```python
from build123d import *
from build123d.topology import SkipClean

# Parameters (mm, degrees)
BOSS_EXTRUDE1_START = 55
SKETCH2_W           = 105
SKETCH2_H           = 22
SKETCH2_R           = 1.8
BOSS_EXTRUDE1_DEPTH = 2
BOSS_EXTRUDE2_START = 2
SKETCH3_R           = 3.8
SKETCH3_R_2         = 1.8
BOSS_EXTRUDE2_DEPTH = 2
BOSS_EXTRUDE3_START = 15
SKETCH5_W           = 105
SKETCH5_H           = 22
SKETCH5_R           = 1.5
BOSS_EXTRUDE3_DEPTH = 2
SKETCH6_W           = 114
SKETCH6_H           = 2
BOSS_EXTRUDE4_DEPTH = 11


with BuildPart() as part:
    # Sketch2 → Boss-Extrude1 (new body)
    with BuildSketch(Plane(origin=(0, 0, 0), x_dir=(0, 0, -1), z_dir=(1, 0, 0)).offset(BOSS_EXTRUDE1_START)):
        Rectangle(SKETCH2_W, SKETCH2_H)
        Circle(SKETCH2_R, mode=Mode.SUBTRACT)
        with Locations((-25.5, 0)):
            Circle(SKETCH2_R, mode=Mode.SUBTRACT)
        with Locations((25.5, 0)):
            Circle(SKETCH2_R, mode=Mode.SUBTRACT)
    extrude(amount=BOSS_EXTRUDE1_DEPTH)

    # Sketch3 → Boss-Extrude2 (add)
    # profile 1 of 2: a face of its own
    with SkipClean():  # the faces are left unmerged after this step: merging them gives an invalid solid
        with BuildSketch(Plane.ZY.offset(-55).offset(BOSS_EXTRUDE2_START)):
            with Locations((-25.5, 0)):
                Circle(SKETCH3_R)
            with Locations((-25.5, 0)):
                Circle(SKETCH3_R_2, mode=Mode.SUBTRACT)
        # profile 2 of 2: a face of its own
        with BuildSketch(Plane.ZY.offset(-55).offset(BOSS_EXTRUDE2_START)):
            with Locations((25.5, 0)):
                Circle(SKETCH3_R)
            with Locations((25.5, 0)):
                Circle(SKETCH3_R_2, mode=Mode.SUBTRACT)
        extrude(amount=-BOSS_EXTRUDE2_DEPTH)


with BuildPart() as body_2:
    # Sketch5 → Boss-Extrude3 (new body)
    with BuildSketch(Plane(origin=(0, 0, 0), x_dir=(0, 0, -1), z_dir=(1, 0, 0)).offset(BOSS_EXTRUDE3_START)):
        Rectangle(SKETCH5_W, SKETCH5_H)
        with Locations((8, 0)):
            Circle(SKETCH5_R, mode=Mode.SUBTRACT)
        with Locations((-8, 0)):
            Circle(SKETCH5_R, mode=Mode.SUBTRACT)
        with Locations((0, 6)):
            Circle(SKETCH5_R, mode=Mode.SUBTRACT)
        with Locations((0, -6)):
            Circle(SKETCH5_R, mode=Mode.SUBTRACT)
    extrude(amount=BOSS_EXTRUDE3_DEPTH)


with BuildPart() as body_3:
    # Mirror2: mirrored copy
    add(part.part.mirror(Plane(origin=(0, 0, 0), x_dir=(0, 0, 1), z_dir=(1, 0, 0))))


with BuildPart() as body_4:
    # Mirror2 2: mirrored copy
    add(body_2.part.mirror(Plane(origin=(0, 0, 0), x_dir=(0, 0, 1), z_dir=(1, 0, 0))))


with BuildPart() as part_1:
    with SkipClean():  # the faces are left unmerged after this step: merging them gives an invalid solid
        add(part.part)

        add(body_2.part)  # Boss-Extrude4 merges body 2

        add(body_3.part)  # Boss-Extrude4 merges body 3

        add(body_4.part)  # Boss-Extrude4 merges body 4
        # Sketch6 → Boss-Extrude4 (add, symmetric)
        with BuildSketch(Plane(origin=(0, 0, 0), x_dir=(1, 0, 0), z_dir=(0, 1, 0))):
            with Locations((0, -51.5)):
                Rectangle(SKETCH6_W, SKETCH6_H)
            with Locations((0, 51.5)):
                Rectangle(SKETCH6_W, SKETCH6_H)
        extrude(amount=BOSS_EXTRUDE4_DEPTH, both=True)


solid = part_1.part
```
Model file for the job. Use its own axes, mm. A direction names the side the tool comes from. Coordinates: 2 decimals unless noted, no trailing zeros. Loops run counter-clockwise (first coordinate to the right, second up) from the corner with the lowest first, then second, coordinate; pieces in that order, holes last. Notation, with made-up numbers: (75.25, 11) - (120.25, 11) arc R27 ccw to (120.25, 42) - close; hole circle Ø8 at (-2.5, 8). An arc over 180 degrees is marked (long way). Answer as a JSON object with one key per item and string values. Group by question number.
(1) Cut at A-A (z = -14.5). Give the cut face in (x, y).
(2) Flat gauge pin, fed straight in: pin 1 (3 mm diameter, centred on y = 0, z = 0, fed in from -X). Where does the tip first touch, or does it go through?
(3) Cut at C-C (z = -25.5). State how many separate pieces and enclosed holes the cut face has, then the cut area to 3 significant figures.
(4) Tool access for faces 1 (the face through (15.99, 0.07, 9.5)), 2 (the face through (15, 0, 1)), 3 (the face through (-16.6, -11, 15.8)): list every direction of +Z, -Z, +X, -X, +Y, -Y with a clear straight run to the whole face (end or side of a thin tool).
(5) Probe line 1 along X through (y, z) = (-2.5, -23.5); line 2 along Y through (x, z) = (-16.25, 0); line 3 along X through (y, z) = (-6, -43). List the from-to ranges inside material, lowest first.
(6) Cut at B-B (x = 33). Give the cut face in (y, z), then the cut area to 3 significant figures.
(7) Two-plate mould, pull along X, no slides. Class faces 4 (the face through (-17, 0, 1)), 5 (the face through (-55.986, 0.541, -1.717)): released by +X, released by -X, zero draft, split by the parting line, or undercut.
(8) Cut at D-D (y = -6). Give the cut face in (x, z), then the cut area to 3 significant figures.
Geometry says:
{
 "1": {"outline": "(-57, -11) - (-55, -11) - (-55, 11) - (-57, 11) - close; (-17, -11) - (-15, -11) - (-15, 11) - (-17, 11) - close; (15, -11) - (17, -11) - (17, 11) - (15, 11) - close; (55, -11) - (57, -11) - (57, 11) - (55, 11) - close"},
 "2": {"pin 1": "stops at x = -17"},
 "3": {"separate pieces": "6", "enclosed holes": "0", "area": "178 mm^2"},
 "4": {"face 1": "none", "face 2": "+Y, -Y", "face 3": "+Z, -Z, +X, -X, -Y"},
 "5": {"line 1": "x = -57 to -53, -17 to -15, 15 to 17, 53 to 57", "line 2": "y = -11 to -7.5, -4.5 to 4.5, 7.5 to 11", "line 3": "x = -57 to -55, -17 to -15, 15 to 17, 55 to 57"},
 "6": {"outline": "(-11, -52.5) - (11, -52.5) - (11, -50.5) - (-11, -50.5) - close; (-11, 50.5) - (11, 50.5) - (11, 52.5) - (-11, 52.5) - close", "area": "88.0 mm^2"},
 "7": {"face 4": "undercut", "face 5": "zero draft"},
 "8": {"outline": "(-57, -52.5) - (57, -52.5) - (57, 52.5) - (-57, 52.5) - close; hole (-55, -50.5) - (-17, -50.5) - (-17, -1.5) - (-15, -1.5) - (-15, -50.5) - (15, -50.5) - (15, -1.5) - (17, -1.5) - (17, -50.5) - (55, -50.5) - (55, 50.5) - (17, 50.5) - (17, 1.5) - (15, 1.5) - (15, 50.5) - (-15, 50.5) - (-15, 1.5) - (-17, 1.5) - (-17, 50.5) - (-55, 50.5) - close", "area": "1,250 mm^2"}
}
